Here's how the part is built. I have some questions about the finished solid (model axes, mm). Coordinates: 2 decimals unless noted, no trailing zeros. Order: outer loops, then holes, each group sorted by start corner. A loop starts at its lowest first (then second) coordinate and runs counter-clockwise, first axis right, second up. Notation, with made-up numbers: (86, 29) - (104, 29) arc R9 cw to (104, 35) - close; hole circle Ø1 at (72, 69). An arc over 180 degrees is marked (long way). Answer as CSV lines item,"result". Start each with the question number.
Q1. I need wall thicknesses on line 1 (Y direction, x = -3, z = 15.5); line 2 (Y direction, x = -8.25, z = 1) (3 decimals); line 3 (Y direction, x = -6.5, z = 13). Which ranges of each line are inside material? Lowest first, please.
Q2. Suppose I cut it at A-A (y = 6.35). Please give me the cut outline in (x, z).
Q3. Suppose I cut it at D-D (z = -25). Please give me the cut outline in (x, y) (3 decimals), then the cut area to 3 significant figures.
Q4. Thinking about a two-plate mould opening in Z: for faces 1 (the face through (-6.409, 4.764, 0.07)), 2 (the face through (-0.493, 18.938, 31.12)), 3 (the face through (-13, 21, 0)), 4 (the face through (-7.86, 40.59, -3.1)), which applies, released by +Z, released by -Z, zero draft, split by the parting line, or undercut?
Q5. Suppose I cut it at B-B (z = 0). Count the separate pieces of the cut face and the enclosed holes in it, then the cut area to 3 significant figures.
Q6. For pin 1 Ø5 at (y, z) = (41.275, 0) entering from -X; pin 2 Ø5 at (x, z) = (-2, 12.5) entering from -Y; pin 3 Ø1.5 at (x, y) = (-8, 36) entering from +Z; pin 4 Ø1.5 at (y, z) = (44.5, -1) entering from +X, each with a flat end and sliding along its axis, tell me the tip position at first contact or that it passes through.
from build123d import *

# Parameters (mm, degrees)
F0_R        = 1.5875
F0_R_2      = 3.175
F1_DEPTH    = 13
F3_DEPTH    = 37.5
F4_R        = 6.35
F5_T1_DEPTH = 88.5
F6_SIZE     = 1
F7_SIZE     = 3.175


# Not quite as in the source:
# - a fillet or chamfer that OpenCascade refuses, or shapes differently, is made with other operations: its cross-section is extruded or revolved along the edge and cut away or added
# - a feature names something its author has since deleted; it is built from what else it names


with BuildPart() as f1:
    # F0 (on Right) → F1 (new body)
    with BuildSketch(Plane.YZ):
        Polygon((0, 31.75), (0, 0), (0, -31.75), (19.05, -31.75), (53.975, -16.7821428571), (53.975, 16.7821428571), (19.05, 31.75), align=None)
        with Locations((9.525, -15.875)):
            Circle(F0_R, mode=Mode.SUBTRACT)
        with Locations((6.35, 0)):
            Circle(F0_R, mode=Mode.SUBTRACT)
        with Locations((9.525, 15.875)):
            Circle(F0_R, mode=Mode.SUBTRACT)
        with Locations((41.275, 0)):
            Circle(F0_R_2, mode=Mode.SUBTRACT)
    extrude(amount=-F1_DEPTH)

    # F2 (on Top) → F3 (cut, symmetric)
    with BuildSketch(Plane.XY):
        with BuildLine():
            Line((0, 30.2764773719), (0, 52.2735226281))
            ThreePointArc((0, 52.2735226281), (-6.35, 41.275), (0, 30.2764773719))
        make_face()
    extrude(amount=F3_DEPTH, both=True, mode=Mode.SUBTRACT)

    # F4
    f4_edges = [f1.edges().sort_by_distance(p)[0] for p in [
        (-6.5, 19.05, 31.75),
        (-6.5, 19.05, -31.75),
        (-6.5, 53.975, 16.782143),
        (-6.5, 53.975, -16.782143),
    ]]
    fillet(f4_edges, radius=F4_R)

    # F5: fillet of radius 5 on 1 edges, made by hand

    # F5_s2 → F5_t1 (cut)
    with BuildSketch(Plane.XY.offset(-44.25)):
        with BuildLine():
            ThreePointArc((0, 5), (-1.4644660941, 1.4644660941), (-5, 0))
            Line((-5, 0), (0, 0))
            Line((0, 0), (0, 5))
        make_face()
    extrude(amount=F5_T1_DEPTH, mode=Mode.SUBTRACT)

    # F6
    f6_edges = [f1.edges().sort_by_distance(p)[0] for p in [
        (0, 11.373307, 31.75),
        (0, 25.262239, -29.087612),
        (0, 25.262239, 29.087612),
        (0, 19.023382, -31.620319),
        (0, 11.373307, -31.75),
        (0, 19.023382, 31.620319),
        (-9, 0, -31.75),
        (-1.464466, 1.464466, -31.75),
        (-1.464466, 1.464466, 31.75),
        (-9, 0, 31.75),
    ]]
    chamfer(f6_edges, length=F6_SIZE)

    # F7
    f7_edges = [f1.edges().sort_by_distance(p)[0] for p in [
        (-13, 38.1, 0),
    ]]
    chamfer(f7_edges, length=F7_SIZE)


solid = f1.part
Here are the results:
1,line 1,"y = 0.42 to 7.98, 11.07 to 32.68, 49.87 to 53.27"
1,line 2,"y = 0 to 5.117, 7.583 to 38.262, 44.288 to 53.975"
1,line 3,"y = 0 to 53.96"
2,outline,"(-13, -31.75) - (-1, -31.75) - (0, -30.75) - (0, -1.59) - (-13, -1.59) - close; (-13, 1.59) - (0, 1.59) - (0, 30.75) - (-1, 31.75) - (-13, 31.75) - close"
3,outline,"(-13, 0) - (-5, 0) arc R5 ccw to (0, 5) - (0, 30.276) arc R12.7 cw to (-4.575, 34.8) - (-13, 34.8) - close"
3,area,"435 mm²"
4,face 1,"undercut"
4,face 2,"released by +Z"
4,face 3,"zero draft"
4,face 4,"undercut"
5,separate pieces,"3"
5,enclosed holes,"0"
5,area,"503 mm²"
6,pin 1,"passes through"
6,pin 2,"stops at y = 0.03"
6,pin 3,"stops at z = 24.81"
6,pin 4,"stops at x = -5.71"
